Input: part model. Units: mm. Frame: model coordinates. Face numbers are marked on the shaded views. A direction names the side the tool comes from. Coordinates: 2 decimals unless noted, no trailing zeros. Write each loop counter-clockwise with the first axis right and the second up, starting at its lowest first coordinate (ties: lowest second). Pieces come first, ordered by that corner, then holes. Notation, with made-up numbers: (14, 46.5) -> (48, 46.5) arc R20 cw to (48, 77.5) -> close; hole circle Ø9 at (-21.5, 69). An arc over 180 degrees is marked (long way). One line per question, with ' | ' between items. Start each with the question number.
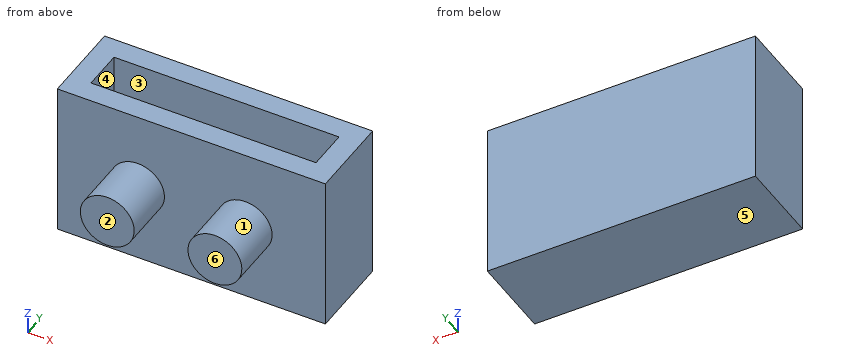
```python
from build123d import *

# Parameters (mm, degrees)
BOSS_EXTRUDE1_DEPTH = 3.8
SKETCH1_3_W         = 20.9
SKETCH1_3_H         = 12.6
BOSS_EXTRUDE2_DEPTH = 2
SKETCH3_R           = 2.5
BOSS_EXTRUDE4_DEPTH = 5
SKETCH4_W           = 24.9
SKETCH4_H           = 14.6
BOSS_EXTRUDE5_DEPTH = 2


with BuildPart() as part:
    # Sketch1 → Boss-Extrude1 (new body)
    with BuildSketch(Plane(origin=(0, 0, 0), x_dir=(1, 0, 0), z_dir=(0, 1, 0))):
        Polygon((22.9, 14.6), (-2, 14.6), (-2, 0), (0, 0), (0, 12.6), (20.9, 12.6), (20.9, 0), (22.9, 0), align=None)
    extrude(amount=BOSS_EXTRUDE1_DEPTH)

    # Sketch1_3 → Boss-Extrude2 (add)
    with BuildSketch(Plane(origin=(0, 0, 0), x_dir=(1, 0, 0), z_dir=(0, 1, 0))):
        with Locations((10.45, 6.3)):
            Rectangle(SKETCH1_3_W, SKETCH1_3_H)
        Polygon((22.9, 14.6), (-2, 14.6), (-2, 0), (0, 0), (0, 12.6), (20.9, 12.6), (20.9, 0), (22.9, 0), align=None)
    extrude(amount=-BOSS_EXTRUDE2_DEPTH)

    # Sketch3 → Boss-Extrude4 (add)
    with BuildSketch(Plane.XZ.offset(2)):
        with Locations(Location((5.45, -7.3, 0), (0, 0, 90))):
            Circle(SKETCH3_R)
        with Locations(Location((15.45, -7.3, 0), (0, 0, 90))):
            Circle(SKETCH3_R)
    extrude(amount=BOSS_EXTRUDE4_DEPTH)

    # Sketch4 → Boss-Extrude5 (add)
    with BuildSketch(Plane(origin=(0, 3.8, 0), x_dir=(1, 0, 0), z_dir=(0, 1, 0))):
        with Locations((10.45, 7.3)):
            Rectangle(SKETCH4_W, SKETCH4_H)
    extrude(amount=BOSS_EXTRUDE5_DEPTH)


solid = part.part
```
1) Section A-A, the plane z = -7.3. Return loops of the section in (x, y).
2) Ray query, line 1 (Y direction, x = 12.75, z = -12); line 2 (X direction, y = 3.75, z = -1.75); line 3 (X direction, y = -2.5, z = -6.25). Return the intervals inside material, ascending.
3) Section C-C, the plane y = -3.75. Return loops of the section in (x, z).
4) Section D-D, the plane y = 0.5. Return loops of the section in (x, z).
5) Pull-direction query (Y, two-part tool) for the marked faces 4, 5 and 6; classes: released by +Y, released by -Y, zero draft, split by the parting line, or undercut.
6) First-contact query: P1, Ø1.5, axis at x = 9.5, z = -4, coming from the -Y side; P2, Ø4, axis at x = 5.5, y = -4.5, coming from the -Z side; P3, Ø1.1, axis at x = 15.5, y = 2.5, coming from the +Z side. Flat tips, straight axial feed; report the tip coordinate or a pass-through.
7) Access query for the marked faces 1, 2 and 3. Directions: +Z, -Z, +X, -X, +Y, -Y. A direction counts if a zero-diameter tool reaches every point of the face in a straight line with its end or side. Return the directions, or none.
8) Section B-B, the plane x = 15.45. Return loops of the section in (y, z), then the cut area to 3 significant figures.
Answer block:
1) outline: (-2, -2) -> (2.95, -2) -> (2.95, -7) -> (7.95, -7) -> (7.95, -2) -> (12.95, -2) -> (12.95, -7) -> (17.95, -7) -> (17.95, -2) -> (22.9, -2) -> (22.9, 5.8) -> (-2, 5.8) -> close; hole (0, 0) -> (20.9, 0) -> (20.9, 3.8) -> (0, 3.8) -> close
2) line 1: y = -2 to 0, 3.8 to 5.8 | line 2: x = -2 to 0, 20.9 to 22.9 | line 3: x = 3.18 to 7.72, 13.18 to 17.72
3) outline: circle Ø5 at (5.45, -7.3); circle Ø5 at (15.45, -7.3)
4) outline: (-2, -14.6) -> (22.9, -14.6) -> (22.9, 0) -> (20.9, 0) -> (20.9, -12.6) -> (0, -12.6) -> (0, 0) -> (-2, 0) -> close
5) face 4: undercut | face 5: zero draft | face 6: released by -Y
6) P1: stops at y = -2 | P2: stops at z = -9.8 | P3: stops at z = -12.6
7) face 1: -Y | face 2: +Z, -Z, +X, -X, -Y | face 3: +Z
8) outline: (-7, -9.8) -> (-2, -9.8) -> (-2, -14.6) -> (5.8, -14.6) -> (5.8, 0) -> (3.8, 0) -> (3.8, -12.6) -> (0, -12.6) -> (0, 0) -> (-2, 0) -> (-2, -4.8) -> (-7, -4.8) -> close | area: 91.0 mm2
